Print and shaded views of the part. All mm, measured from the part's lowest x, y and z. Round coordinates to 2 decimals unless told otherwise and drop trailing zeros. Order: outer loops, then holes, each group sorted by start corner. A loop starts at its lowest first (then second) coordinate and runs counter-clockwise, first axis right, second up. Notation, with made-up numbers: (76.5, -4) - (97.5, -4) arc R24 cw to (97.5, 19) - close; hole circle Ø2 at (19, 44.5). An arc over 180 degrees is marked (long way). Write item = value, one per line.
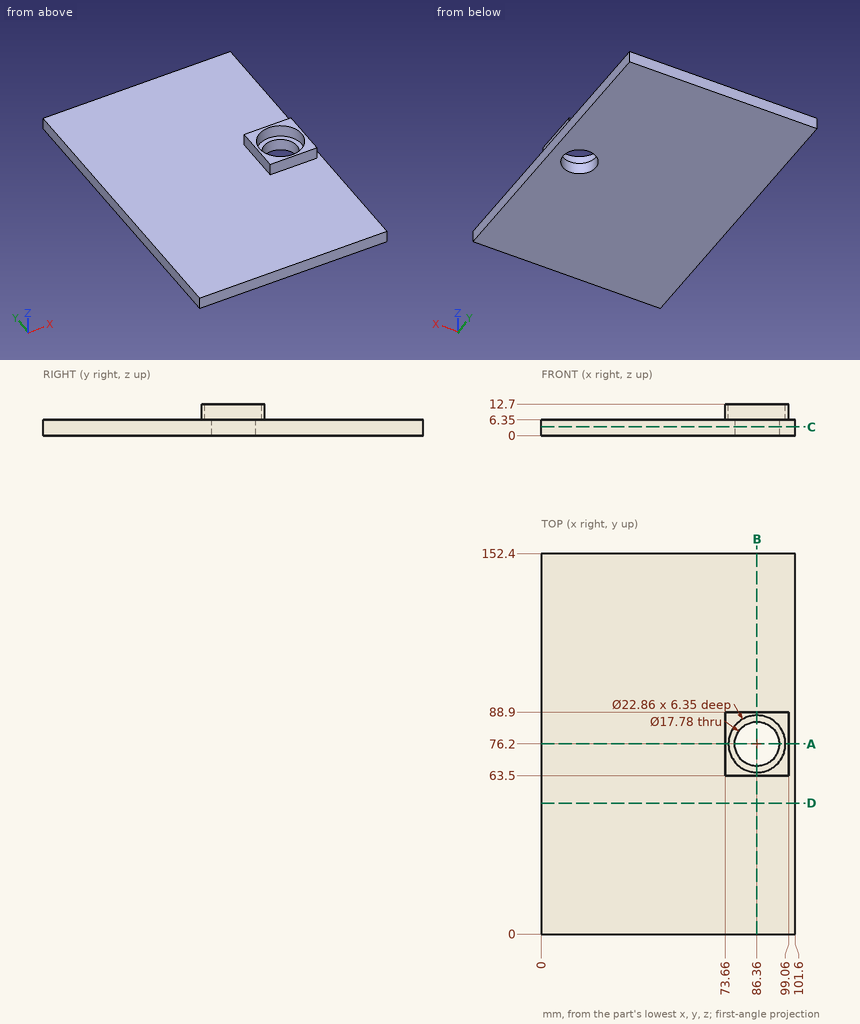
(1) Drop flat-ended pins along their axis: pin 1 (1.9 mm diameter, centred on y = 75.5, z = 11, fed in from -X); pin 2 (4 mm diameter, centred on x = 19, y = 40.5, fed in from +Z); pin 3 (1.9 mm diameter, centred on x = 88.5, z = 11, fed in from -Y). Give the stop position or say it passes through.
Solved:
pin_1 = 73.66
pin_2 = 6.35
pin_3 = 63.5
(2) Band-saw the part on A-A on y = 76.2. List the corners of the cut face in (x, z), plus the area to 3 significant figures.
Solved:
outline = (0, 0) - (77.47, 0) - (77.47, 6.35) - (74.93, 6.35) - (74.93, 12.7) - (73.66, 12.7) - (73.66, 6.35) - (0, 6.35) - close; (95.25, 0) - (101.6, 0) - (101.6, 6.35) - (99.06, 6.35) - (99.06, 12.7) - (97.79, 12.7) - (97.79, 6.35) - (95.25, 6.35) - close
area = 548 mm²
(3) Probe line 1 along Y through (x, z) = (86.36, 2); line 2 along Y through (x, z) = (86.36, 8.75); line 3 along Z through (x, y) = (59.5, 65.5). List the from-to ranges inside material, lowest first.
Solved:
line_1 = 0 to 67.31, 85.09 to 152.4
line_2 = 63.5 to 64.77, 87.63 to 88.9
line_3 = 0 to 6.35
(4) Band-saw the part on B-B on x = 86.36. List the corners of the cut face in (y, z).
Solved:
outline = (0, 0) - (67.31, 0) - (67.31, 6.35) - (64.77, 6.35) - (64.77, 12.7) - (63.5, 12.7) - (63.5, 6.35) - (0, 6.35) - close; (85.09, 0) - (152.4, 0) - (152.4, 6.35) - (88.9, 6.35) - (88.9, 12.7) - (87.63, 12.7) - (87.63, 6.35) - (85.09, 6.35) - close
(5) Band-saw the part on D-D on y = 52.5. List the corners of the cut face in (x, z).
Solved:
outline = (0, 0) - (101.6, 0) - (101.6, 6.35) - (0, 6.35) - close
(6) Band-saw the part on C-C on z = 3.5. List the corners of the cut face in (x, y).
Solved:
outline = (0, 0) - (101.6, 0) - (101.6, 152.4) - (0, 152.4) - close; hole circle Ø17.78 at (86.36, 76.2)
